Read the model definition and answer for the solid it produces. Units are mm, in the model's axes. A direction names the side the tool comes from. Round coordinates to 2 decimals unless told otherwise and drop trailing zeros. Loops run counter-clockwise (first coordinate to the right, second up) from the corner with the lowest first, then second, coordinate; pieces in that order, holes last. Notation, with made-up numbers: M 50.25,78 L 94.25,78 A13 cw 94.25,98 Z; hole C 55,12.5 d7. An arc over 180 degrees is marked long. Write each question's results on one line, items separated by ' | '.
```python
from build123d import *

# Parameters (mm, degrees)
ESQUISSE1_R                  = 34.5
BOSS_EXTRU_1_DEPTH           = 3
ESQUISSE2_R                  = 34.5
ESQUISSE2_R_2                = 31.7
BOSS_EXTRU_2_DEPTH           = 15
ENL_V_MAT_EXTRU_1_DEPTH      = 53.00480747
ENL_V_MAT_EXTRU_1_DEPTH_BACK = 53.00480747
ESQUISSE3_R                  = 13.5
CONG_1_R                     = 2


with BuildPart() as part:
    # Esquisse1 → Boss.-Extru.1 (new body)
    with BuildSketch(Plane.XY):
        Circle(ESQUISSE1_R)
    extrude(amount=BOSS_EXTRU_1_DEPTH)

    # Esquisse2 → Boss.-Extru.2 (add)
    with BuildSketch(Plane.XY.offset(3)):
        Circle(ESQUISSE2_R)
        Circle(ESQUISSE2_R_2, mode=Mode.SUBTRACT)
    extrude(amount=BOSS_EXTRU_2_DEPTH)

    # Esquisse3 → Enlèv. mat.-Extru.1 (cut, two sides: drawn at the far end of the back side and taken through both)
    with BuildSketch(Plane(origin=(0, 0, 0), x_dir=(-1, 0, 0), z_dir=(0, 0, -1)).offset(-ENL_V_MAT_EXTRU_1_DEPTH_BACK)):
        with Locations(Location((0, 0, 0), (0, 0, 180))):
            Circle(ESQUISSE3_R)
    extrude(amount=ENL_V_MAT_EXTRU_1_DEPTH + ENL_V_MAT_EXTRU_1_DEPTH_BACK, mode=Mode.SUBTRACT)

    # Congé1
    cong_1_edges = [part.edges().sort_by_distance(p)[0] for p in [
        (-34.5, 0, 0),
    ]]
    fillet(cong_1_edges, radius=CONG_1_R)


solid = part.part
```
1. Given P1, Ø3, axis at y = 3, z = 2.5, coming from the -X side; P2, Ø1, axis at y = -3.5, z = 10, coming from the -X side; P3, Ø1, axis at y = -16.5, z = 10.5, coming from the -X side; P4, Ø24.5, axis at x = 0, y = 0, coming from the +Z side, each flat-ended and moving along its own axis, determine where each tip first touches the part or whether it passes through.
Completed:
P1: stops at x = -34.47 | P2: stops at x = -34.37 | P3: stops at x = -30.57 | P4: passes through
2. Find section A-A, the plane y = 0. Give the vertices of the cut face in (x, z), then the cut area to 3 significant figures.
Completed:
outline: M -34.5,2 A2 ccw -32.5,0 L -13.5,0 L -13.5,3 L -31.7,3 L -31.7,18 L -34.5,18 Z; M 13.5,0 L 32.5,0 A2 ccw 34.5,2 L 34.5,18 L 31.7,18 L 31.7,3 L 13.5,3 Z | area: 208 mm2
3. Determine the mould class of faces 1 (the face through (15.2, -28, 18)), 2 (the face through (14, 0, 3)), 3 (the face through (32.907, 10.363, 9.888)) for opening direction X: released by +X, released by -X, zero draft, split by the parting line, or undercut.
Completed:
face 1: zero draft | face 2: undercut | face 3: split by the parting line
4. Find section C-C, the plane z = 6.5. Give the vertices of the cut face in (x, y).
Completed:
outline: C 0,0 d69; hole C 0,0 d63.4
5. Which of the six approach directions +Z, -Z, +X, -X, +Y, -Y give full straight-line access (tool end or side, diameter ignored) to faces 4 (the face through (-2.93, 13.18, 1.52)), 5 (the face through (30.236, 9.522, 10.395))?
Completed:
face 4: +Z, -Z | face 5: +Z
6. Find the intervals of material crossed by L1, parallel to Y at x = 0, z = 2.2; L2, parallel to Y at x = 0, z = 9.5; L3, parallel to Z at x = 9, y = -11, in increasing order.
Completed:
L1: y = -34.5 to -13.5, 13.5 to 34.5 | L2: y = -34.5 to -31.7, 31.7 to 34.5 | L3: z = 0 to 3
